from build123d import *

# Parameters (mm, degrees)
SKETCH1_R           = 12.5
BOSS_EXTRUDE1_DEPTH = 9
SKETCH2_R           = 10
BOSS_EXTRUDE2_DEPTH = 7.6
SKETCH3_R           = 12.5
BOSS_EXTRUDE3_DEPTH = 1.5
SKETCH4_R           = 2.5
CUT_EXTRUDE1_DEPTH  = 19.1


with BuildPart() as part:
    # Sketch1 → Boss-Extrude1 (new body)
    with BuildSketch(Plane(origin=(0, 0, 0), x_dir=(1, 0, 0), z_dir=(0, 1, 0))):
        Circle(SKETCH1_R)
    extrude(amount=BOSS_EXTRUDE1_DEPTH)

    # Sketch2 → Boss-Extrude2 (add)
    with BuildSketch(Plane(origin=(0, 9, 0), x_dir=(1, 0, 0), z_dir=(0, 1, 0))):
        Circle(SKETCH2_R)
    extrude(amount=BOSS_EXTRUDE2_DEPTH)

    # Sketch3 → Boss-Extrude3 (add)
    with BuildSketch(Plane(origin=(0, 16.6, 0), x_dir=(1, 0, 0), z_dir=(0, 1, 0))):
        Circle(SKETCH3_R)
    extrude(amount=BOSS_EXTRUDE3_DEPTH)

    # Sketch4 → Cut-Extrude1 (cut, through all)
    with BuildSketch(Plane(origin=(0, 18.1, 0), x_dir=(1, 0, 0), z_dir=(0, 1, 0))):
        Circle(SKETCH4_R)
    extrude(amount=-CUT_EXTRUDE1_DEPTH, mode=Mode.SUBTRACT)


solid = part.part
Source: CAD feature listing. Evaluate the final solid. Frame: model axes, mm. A direction names the side the tool comes from. Give positions to 0.01 mm unless a question says otherwise; leave off trailing zeros. Write each loop counter-clockwise with the first axis right and the second up, starting at its lowest first coordinate (ties: lowest second). Pieces come first, ordered by that corner, then holes. Notation, with made-up numbers: (24.5, 83) -> (69.5, 83) arc R26 cw to (69.5, 103) -> close; hole circle Ø6 at (16, 14). An arc over 180 degrees is marked (long way). Return JSON: item names as keys, results as strings. Group by question number.
1. Section B-B, the plane z = 0. Output: boundary loops of the cut face in (x, y).
2. Section C-C, the plane y = 8.5. Output: boundary loops of the cut face in (x, z), then the cut area to 3 significant figures.
3. Section A-A, the plane x = 0. Output: boundary loops of the cut face in (y, z), then the cut area to 3 significant figures.
4. Pin query (flat end, axial travel): pin 1 Ø2 at (y, z) = (12.5, -4.5) entering from -X; pin 2 Ø10 at (x, y) = (7.5, 2.5) entering from -Z; pin 3 Ø1.5 at (x, y) = (4.5, 3) entering from -Z. Return the tip coordinate at first contact, or that it passes through.
5. Material intervals for line 1 (X direction, y = 4, z = 0); line 2 (Y direction, x = -4, z = -9.25); line 3 (Z direction, x = 0, y = 12.75), sorted ascending. Write a range as from..to.
6. Mould query, pull axis Y, two halves, no side actions, for faces 1 (the face through (0, 18.1, 3)), 2 (the face through (11.923, 17.34, -3.755)), 3 (the face through (0, 0, 3)), 4 (the face through (-0.1, 16.6, -10.2)). Classes: +Y half, -Y half, draft (parallel to the pull), parting line (faces both ways), or undercut.
7. Section D-D, the plane x = -5.25. Output: boundary loops of the cut face in (y, z).
8. Access query for faces 5 (the face through (11.923, 4.437, -3.755)), 6 (the face through (-2.17, 12.75, 9.76)). Directions: +Z, -Z, +X, -X, +Y, -Y. A direction counts if a zero-diameter tool reaches every point of the face in a straight line with its end or side. Return the directions, or none.
Determined:
{
 "1": {"outline": "(-12.5, 0) -> (-2.5, 0) -> (-2.5, 18.1) -> (-12.5, 18.1) -> (-12.5, 16.6) -> (-10, 16.6) -> (-10, 9) -> (-12.5, 9) -> close; (2.5, 0) -> (12.5, 0) -> (12.5, 9) -> (10, 9) -> (10, 16.6) -> (12.5, 16.6) -> (12.5, 18.1) -> (2.5, 18.1) -> close"},
 "2": {"outline": "circle Ø25 at (0, 0); hole circle Ø5 at (0, 0)", "area": "471 mm2"},
 "3": {"outline": "(0, -12.5) -> (9, -12.5) -> (9, -10) -> (16.6, -10) -> (16.6, -12.5) -> (18.1, -12.5) -> (18.1, -2.5) -> (0, -2.5) -> close; (0, 2.5) -> (18.1, 2.5) -> (18.1, 12.5) -> (16.6, 12.5) -> (16.6, 10) -> (9, 10) -> (9, 12.5) -> (0, 12.5) -> close", "area": "324 mm2"},
 "4": {"pin 1": "stops at x = -9.37", "pin 2": "stops at z = -12.25", "pin 3": "stops at z = -11.92"},
 "5": {"line 1": "x = -12.5..-2.5, 2.5..12.5", "line 2": "y = 0..9, 16.6..18.1", "line 3": "z = -10..-2.5, 2.5..10"},
 "6": {"face 1": "+Y half", "face 2": "draft", "face 3": "-Y half", "face 4": "undercut"},
 "7": {"outline": "(0, -11.34) -> (9, -11.34) -> (9, -8.51) -> (16.6, -8.51) -> (16.6, -11.34) -> (18.1, -11.34) -> (18.1, 11.34) -> (16.6, 11.34) -> (16.6, 8.51) -> (9, 8.51) -> (9, 11.34) -> (0, 11.34) -> close"},
 "8": {"face 5": "+Y, -Y", "face 6": "none"}
}
